Read the model definition and answer for the solid it produces. Units are mm, in the model's axes. Face numbers are marked on the shaded views. A direction names the side the tool comes from. Give positions to 0.01 mm unless a question says otherwise; leave off trailing zeros. Order: outer loops, then holes, each group sorted by start corner. A loop starts at its lowest first (then second) coordinate and runs counter-clockwise, first axis right, second up. Notation, with made-up numbers: M -33,78 L -25,78 A27 ccw -25,111 Z; hole C -5.75,70.5 d5. An arc over 180 degrees is marked long. Write item = value, one per line. Start each with the question number.
from build123d import *


with BuildPart() as part:
    # Szkic1 → Obrót1 (revolve)
    with BuildSketch(Plane.XY, mode=Mode.PRIVATE) as obr_t1_sk:
        with BuildLine():
            Line((0.901941932, 8.019611614), (-8.880388386, 9.976077677))
            ThreePointArc((-8.880388386, 9.976077677), (-8.963398891, 9.955353824), (-9, 9.87801961))
            Line((-9, 9.87801961), (-9, 7.58198039))
            ThreePointArc((-9, 7.58198039), (-8.977334214, 7.5185815), (-8.919611614, 7.483922323))
            Line((-8.919611614, 7.483922323), (-1.645644932, 6.029128986))
            Line((-1.645644932, 6.029128986), (-1.645644932, -0.5))
            Line((-1.645644932, -0.5), (0, -0.5))
            Line((0, -0.5), (0, 2))
            ThreePointArc((0, 2), (0.146446609, 2.353553391), (0.5, 2.5))
            Line((0.5, 2.5), (1, 2.5))
            Line((1, 2.5), (1, 5.5))
            Line((1, 5.5), (0.5, 5.5))
            Line((0.5, 5.5), (0.980388386, 7.901941932))
            ThreePointArc((0.980388386, 7.901941932), (0.965535348, 7.977023566), (0.901941932, 8.019611614))
        make_face()
    revolve(obr_t1_sk.sketch.rotate(Axis((0, -11.7, 0), (-1, 0, 0)), 90), axis=Axis((0, -11.7, 0), (-1, 0, 0)))


solid = part.part
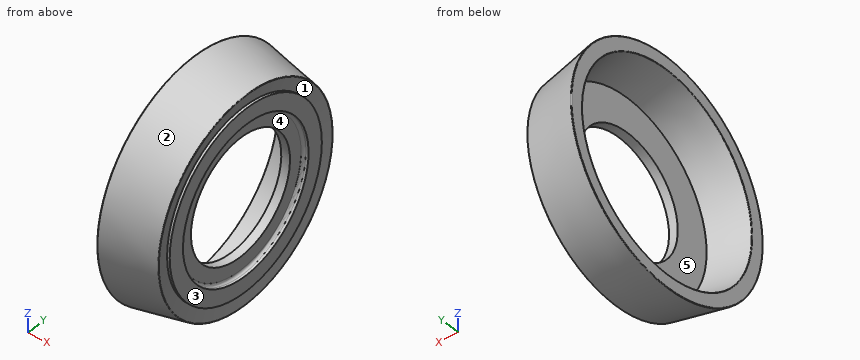
1) Each of these flat-tipped pins is pushed along its axis until it touches: P1, Ø8, axis at y = -12.5, z = -11, coming from the -X side; P2, Ø13.5, axis at y = -15, z = 2.5, coming from the +X side; P3, Ø2, axis at x = -6, z = -4, coming from the -Y side; P4, Ø2, axis at x = -6, y = -25.5, coming from the -Z side. Where does it stop, or does it pass through?
2) Find section B-B on z = 0. Determine the outline of the cut face in (x, y), plus the area to 3 significant figures.
3) Find section C-C on x = -5. Determine the outline of the cut face in (y, z).
4) For the marked faces 4 and 5, determine the directions among +Z, -Z, +X, -X, +Y, -Y from which every point of the face is accessible in a straight line to the end or side of a thin tool.
5) Find section D-D on x = -8. Determine the outline of the cut face in (y, z), plus the area to 3 significant figures.
6) For a pull along Y with two mould halves and no side action, classify the marked faces 1, 2 and 3 as pulls with the +Y half, pulls with the -Y half, needs draft (parallel to the pull), parting line crosses it, or undercut.
7) Find section A-A on y = -11.7. Determine the outline of the cut face in (x, z).
8) Find the intervals of material crossed by probe 1 along X at (y, z) = (0.5, 1); probe 2 along Y at (x, z) = (-2.75, -14); probe 3 along Z at (x, y) = (-5.25, -22), in increasing order. Write a range as [from, to].
Numbers:
q1.P1 = -1.65
q1.P2 = through
q1.P3 = -32.69
q1.P4 = -16.81
q2.outline = M -9,-33.28 A0.1 ccw -8.88,-33.38 L 0.9,-31.42 A0.1 ccw 0.98,-31.3 L 0.5,-28.9 L 1,-28.9 L 1,-25.9 L 0.5,-25.9 A0.5 cw 0,-25.4 L 0,-22.9 L -1.65,-22.9 L -1.65,-29.43 L -8.92,-30.88 A0.1 ccw -9,-30.98 Z; M -9,7.58 A0.1 ccw -8.92,7.48 L -1.65,6.03 L -1.65,-0.5 L 0,-0.5 L 0,2 A0.5 cw 0.5,2.5 L 1,2.5 L 1,5.5 L 0.5,5.5 L 0.98,7.9 A0.1 ccw 0.9,8.02 L -8.88,9.98 A0.1 ccw -9,9.88 Z
q2.area = 76.0 mm2
q3.outline = C -11.7,0 d41.8; hole C -11.7,0 d36.8
q4.face_4 = +X
q4.face_5 = -X
q5.outline = C -11.7,0 d43; hole C -11.7,0 d38
q5.area = 318 mm2
q6.face_1 = undercut
q6.face_2 = parting line crosses it
q6.face_3 = needs draft
q7.outline = M -9,-21.58 A0.1 ccw -8.88,-21.68 L 0.9,-19.72 A0.1 ccw 0.98,-19.6 L 0.5,-17.2 L 1,-17.2 L 1,-14.2 L 0.5,-14.2 A0.5 cw 0,-13.7 L 0,-11.2 L -1.65,-11.2 L -1.65,-17.73 L -8.92,-19.18 A0.1 ccw -9,-19.28 Z; M -9,19.28 A0.1 ccw -8.92,19.18 L -1.65,17.73 L -1.65,11.2 L 0,11.2 L 0,13.7 A0.5 cw 0.5,14.2 L 1,14.2 L 1,17.2 L 0.5,17.2 L 0.98,19.6 A0.1 ccw 0.9,19.72 L -8.88,21.68 A0.1 ccw -9,21.58 Z
q8.probe_1 = [-1.65, 0]
q8.probe_2 = [-26.61, -22.93], [-0.47, 3.21]
q8.probe_3 = [-18.24, -15.31], [15.31, 18.24]
